Source: CAD feature listing. Evaluate the final solid. Frame: model axes, mm. Face numbers are marked on the shaded views. Give positions to 0.01 mm unless a question says otherwise; leave off trailing zeros. Write each loop counter-clockwise with the first axis right and the second up, starting at its lowest first coordinate (ties: lowest second). Pieces come first, ordered by that corner, then holes. Notation, with made-up numbers: (28, 9.5) -> (52, 9.5) arc R29 cw to (52, 36.5) -> close; hole circle Ø9 at (86, 22.5). An arc over 180 degrees is marked (long way). Use a Markdown table: item, result. Add a question column.
```python
from build123d import *

# Parameters (mm, degrees)
MODEL_R         = 1
MODEL_R_2       = 2.5
EXTRUDE_1_DEPTH = 1.2


with BuildPart() as part:
    # Model → 凸台-拉伸1 (new body)
    with BuildSketch(Plane.XY):
        with BuildLine():
            ThreePointArc((12.485683382, 19.826470809), (12.652302696, 19.686300725), (12.828649886, 19.55858496))
            ThreePointArc((12.828649886, 19.55858496), (15.184787498, 18.84198425), (17.540925109, 19.55858496))
            ThreePointArc((17.540925109, 19.55858496), (17.7172723, 19.686300725), (17.883891613, 19.826470809))
            ThreePointArc((17.883891613, 19.826470809), (21.053773782, 19.747678625), (21.132565966, 16.577796457))
            ThreePointArc((21.132565966, 16.577796457), (20.992395882, 16.411177143), (20.864680117, 16.234829953))
            ThreePointArc((20.864680117, 16.234829953), (20.148079407, 13.878692341), (20.864680117, 11.522554729))
            ThreePointArc((20.864680117, 11.522554729), (20.992395882, 11.346207539), (21.132565966, 11.179588225))
            ThreePointArc((21.132565966, 11.179588225), (21.053773782, 8.009706057), (17.883891613, 7.930913873))
            ThreePointArc((17.883891613, 7.930913873), (17.7172723, 8.071083957), (17.540925109, 8.198799722))
            ThreePointArc((17.540925109, 8.198799722), (15.184787498, 8.915400432), (12.828649886, 8.198799722))
            ThreePointArc((12.828649886, 8.198799722), (12.652302696, 8.071083957), (12.485683382, 7.930913873))
            ThreePointArc((12.485683382, 7.930913873), (9.315801214, 8.009706057), (9.237009029, 11.179588225))
            ThreePointArc((9.237009029, 11.179588225), (9.377179113, 11.346207539), (9.504894878, 11.522554729))
            ThreePointArc((9.504894878, 11.522554729), (10.221495588, 13.878692341), (9.504894878, 16.234829953))
            ThreePointArc((9.504894878, 16.234829953), (9.377179113, 16.411177143), (9.237009029, 16.577796457))
            ThreePointArc((9.237009029, 16.577796457), (9.315801214, 19.747678625), (12.485683382, 19.826470809))
        make_face()
        with Locations((18.296057335, 16.989962178)):
            Circle(MODEL_R, mode=Mode.SUBTRACT)
        with Locations((12.07351766, 16.989962178)):
            Circle(MODEL_R, mode=Mode.SUBTRACT)
        with Locations((12.07351766, 10.767422504)):
            Circle(MODEL_R, mode=Mode.SUBTRACT)
        with Locations((18.296057335, 10.767422504)):
            Circle(MODEL_R, mode=Mode.SUBTRACT)
        with Locations((15.184787498, 13.878692341)):
            Circle(MODEL_R_2, mode=Mode.SUBTRACT)
    extrude(amount=EXTRUDE_1_DEPTH)


solid = part.part
```
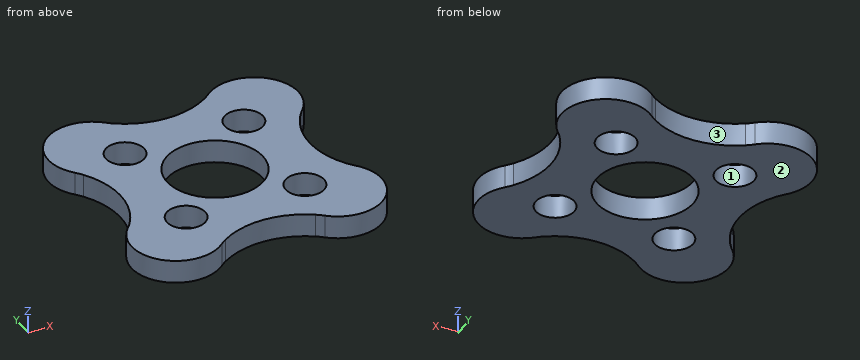
(1) Cut plane D-D on z = 0.25. Return the cut outline in (x, y), then the cut area to 3 significant figures.
(2) Cut plane B-B on y = 8.75. Return the cut outline in (x, z).
(3) Cut plane C-C on x = 19. Return the cut outline in (y, z), then the cut area to 3 significant figures.
(4) Material intervals for L1, parallel to Y at x = 11.5, z = 1.05; L2, parallel to X at y = 10, z = 0.6; L3, parallel to Y at x = 19, z = 1.05, sorted ascending.
(5) Mould query, pull axis Y, two halves, no side actions, for the marked faces 1, 2 and 3. Classes: +Y half, -Y half, draft (parallel to the pull), parting line (faces both ways), or undercut.
(6) Cut plane A-A on x = 14. Return the cut outline in (y, z).
Output:
| question | item | result |
|---|---|---|
| 1 | outline | (9.24, 11.18) arc R2.3 ccw to (12.49, 7.93) arc R3 cw to (12.83, 8.2) arc R4.23 cw to (17.54, 8.2) arc R3 cw to (17.88, 7.93) arc R2.3 ccw to (21.13, 11.18) arc R3 cw to (20.86, 11.52) arc R4.23 cw to (20.86, 16.23) arc R3 cw to (21.13, 16.58) arc R2.3 ccw to (17.88, 19.83) arc R3 cw to (17.54, 19.56) arc R4.23 cw to (12.83, 19.56) arc R3 cw to (12.49, 19.83) arc R2.3 ccw to (9.24, 16.58) arc R3 cw to (9.5, 16.23) arc R4.23 cw to (9.5, 11.52) arc R3 cw to start; hole circle Ø2 at (12.07, 10.77); hole circle Ø2 at (12.07, 16.99); hole circle Ø5 at (15.18, 13.88); hole circle Ø2 at (18.3, 10.77); hole circle Ø2 at (18.3, 16.99) |
| 1 | area | 105 mm^2 |
| 2 | outline | (8.82, 0) -> (14.01, 0) -> (14.01, 1.2) -> (8.82, 1.2) -> close; (16.36, 0) -> (21.55, 0) -> (21.55, 1.2) -> (16.36, 1.2) -> close |
| 3 | outline | (7.38, 0) -> (10.06, 0) -> (10.06, 1.2) -> (7.38, 1.2) -> close; (11.48, 0) -> (16.28, 0) -> (16.28, 1.2) -> (11.48, 1.2) -> close; (17.7, 0) -> (20.38, 0) -> (20.38, 1.2) -> (17.7, 1.2) -> close |
| 3 | area | 12.2 mm^2 |
| 4 | L1 | 7.4 to 9.95, 11.59 to 16.17, 17.81 to 20.35 |
| 4 | L2 | 8.67 to 11.43, 12.71 to 17.65, 18.94 to 21.7 |
| 4 | L3 | 7.38 to 10.06, 11.48 to 16.28, 17.7 to 20.38 |
| 5 | face 1 | undercut |
| 5 | face 2 | draft |
| 5 | face 3 | +Y half |
| 6 | outline | (8.75, 0) -> (11.68, 0) -> (11.68, 1.2) -> (8.75, 1.2) -> close; (16.08, 0) -> (19.01, 0) -> (19.01, 1.2) -> (16.08, 1.2) -> close |
